Here's how the part is built. I have some questions about the finished solid (model axes, mm). A direction names the side the tool comes from. Round coordinates to 2 decimals unless told otherwise and drop trailing zeros. Loops run counter-clockwise (first coordinate to the right, second up) from the corner with the lowest first, then second, coordinate; pieces in that order, holes last. Notation, with made-up numbers: M 17,-33.75 L 55,-33.75 A11 cw 55,-14.75 Z; hole C 32.5,50 d10. An arc over 180 degrees is marked long. Write each question's results on one line, items separated by ' | '. Start each with the question number.
```python
from build123d import *

# Parameters (mm, degrees)
F0_R      = 100
F1_DEPTH  = 25
F2_R      = 5
F3_R      = 90
F4_DEPTH  = 150
F6_DEPTH  = 300.001
F7_W      = 25
F7_H      = 200
F8_DEPTH  = 1
F10_W     = 180
F10_H     = 18.838352
F11_DEPTH = 1


with BuildPart() as f1:
    # F0 (on Top) → F1 (new body)
    with BuildSketch(Plane.XY):
        with BuildLine():
            ThreePointArc((-150, -150), (-120.710678, -220.710678), (-50, -250))
            Line((-50, -250), (50, -250))
            ThreePointArc((50, -250), (120.710678, -220.710678), (150, -150))
            Line((150, -150), (150, 250))
            Line((150, 250), (-150, 250))
            Line((-150, 250), (-150, -150))
        make_face()
        with Locations((0, -40)):
            Circle(F0_R, mode=Mode.SUBTRACT)
    extrude(amount=-F1_DEPTH)

    # F2
    f2_edges = [f1.edges().sort_by_distance(p)[0] for p in [
        (150, 250, -12.5),
        (-150, 250, -12.5),
    ]]
    fillet(f2_edges, radius=F2_R)

    # F3 (on face) → F4 (join)
    with BuildSketch(Plane(origin=(0, 250, 0), x_dir=(-1, 0, 0), z_dir=(0, 1, 0))):
        with BuildLine():
            ThreePointArc((-99.979435, 97.972075), (1.014014, 0.005141), (100, 100))
            ThreePointArc((100, 100), (-1.014014, 199.994859), (-99.979435, 97.972075))
        make_face()
        with Locations((0, 100)):
            Circle(F3_R, mode=Mode.SUBTRACT)
        with BuildLine():
            ThreePointArc((0, 0), (-69.990026, 28.575941), (-99.979435, 97.972075))
            Line((-99.979435, 97.972075), (-145, 0))
            Line((-145, 0), (0, 0))
        make_face()
        with BuildLine():
            Line((145, 0), (100, 100))
            ThreePointArc((100, 100), (70.710678, 29.289322), (0, 0))
            Line((0, 0), (145, 0))
        make_face()
    extrude(amount=-F4_DEPTH)

    # F5 (on face) → F6 (cut, through all)
    with BuildSketch(Plane.YZ.offset(150)):
        Polygon((98.237798, 200.659841), (98.237798, 0), (148.237798, 200.659841), align=None)
    extrude(amount=-F6_DEPTH, mode=Mode.SUBTRACT)

    # F7 (on face) → F8 (join)
    with BuildSketch(Plane.XY):
        with Locations((0, -40)):
            Rectangle(F7_W, F7_H)
    extrude(amount=-F8_DEPTH)

    # F10 (on offset) → F11 (join)
    with BuildSketch(Plane.XZ.offset(-150)):
        with Locations((0, 100)):
            Rectangle(F10_W, F10_H)
    extrude(amount=F11_DEPTH)


solid = f1.part
```
Item 1: If we section it at C-C on x = -34: Please give me the cut outline in (y, z), and give its area (3 significant figures).
Item 2: If we mould it in two halves opening along X, with no side actions, what happens to faces 1 (the face through (-122.815, 176.05, 49.3)), 2 (the face through (-1, 150, 100)), 3 (the face through (-1, 149, 100)), 4 (the face through (122.175, 176.05, 49.672))? For each: released by +X, released by -X, zero draft, split by the parting line, or undercut.
Item 3: I'm going to push flat-ended pins straight in: pin 1 (1.5 mm diameter, centred on x = -108.5, y = -94, fed in from +Z); pin 2 (3.5 mm diameter, centred on x = -13, z = 2, fed in from -Y); pin 3 (12 mm diameter, centred on y = 132, z = 95, fed in from -X). Where does each tip first touch, or does it pass through?
Item 4: If we section it at B-B on z = 114.5: Please give me the cut outline in (x, y).
Item 5: If we section it at D-D on x = 0: Please give me the cut outline in (y, z).
Item 6: Which directions (+Z, -Z, +X, -X, +Y, -Y) give clear straight access to the entire face, cutting with the end or side of a thin tool? Please do faces 5 (the face through (-1, -250, -12)), 6 (the face through (0, -39, -1)).
Item 7: I need wall thicknesses on L1, parallel to X at y = -40, z = -6; L2, parallel to Z at x = 0, y = 201.5; L3, parallel to Y at x = 0, z = -11. Which ranges of each line are inside material? Lowest first, please.
Item 8: If we section it at A-A on y = -40: Please give me the cut outline in (x, z), and give its area (4 significant figures).
Numbers:
1) outline: M -250,-25 L -134.04,-25 L -134.04,0 L -250,0 Z; M 54.04,-25 L 250,-25 L 250,16.67 L 102.39,16.67 L 100,7.07 L 100,0 L 54.04,0 Z; M 143.92,183.33 L 250,183.33 L 250,194.04 L 146.59,194.04 Z; M 149,90.58 L 150,90.58 L 150,109.42 L 149,109.42 Z | area: 11,400 mm²
2) face 1: released by -X | face 2: undercut | face 3: undercut | face 4: released by +X
3) pin 1: z = 0 | pin 2: y = 100 | pin 3: x = -104.95
4) outline: M -98.94,126.77 L -88.82,126.77 L -88.82,250 L -98.94,250 Z; M 88.82,126.77 L 98.94,126.77 L 98.94,250 L 88.82,250 Z
5) outline: M -250,-25 L -140,-25 L -140,-1 L 60,-1 L 60,-25 L 250,-25 L 250,10 L 100.73,10 L 100,7.07 L 100,0 L -250,0 Z; M 145.58,190 L 250,190 L 250,200 L 148.07,200 Z; M 149,90.58 L 150,90.58 L 150,109.42 L 149,109.42 Z
6) face 5: +Z, -Z, +X, -X, -Y | face 6: -Z
7) L1: -150 to -100, 100 to 150 | L2: -25 to 10, 190 to 200 | L3: -250 to -140, 60 to 250
8) outline: M -150,-25 L -100,-25 L -100,0 L -150,0 Z; M -12.5,-1 L 12.5,-1 L 12.5,0 L -12.5,0 Z; M 100,-25 L 150,-25 L 150,0 L 100,0 Z | area: 2,525 mm²
